from build123d import *

# Parameters (mm, degrees)
PAD018_DEPTH    = 8.5
FILLET008_R     = 6
FILLET009_R     = 3
SKETCH032_R     = 84.3
POCKET021_DEPTH = 9.6
SKETCH033_R     = 1
POCKET022_DEPTH = 17.001
FILLET010_R     = 6


with BuildPart() as part:
    # Sketch031 → Pad018 (new body, symmetric)
    with BuildSketch(Plane.XY):
        with BuildLine():
            Line((226.925203, 42.33455), (276.925203, 128.93709))
            ThreePointArc((310.700194, 109.43709), (294.5, 120.377531), (276.925203, 128.93709))
            Line((260.700194, 22.83455), (310.700194, 109.43709))
            Line((226.925203, 42.33455), (260.700194, 22.83455))
        make_face()
        with BuildLine():
            Line((259.708266, 93.11648), (278.208266, 125.15942))
            ThreePointArc((306.787104, 108.65942), (293, 117.779455), (278.208266, 125.15942))
            Line((288.287104, 76.61648), (306.787104, 108.65942))
            ThreePointArc((288.287104, 76.61648), (274.687379, 86.061065), (259.708266, 93.11648))
        make_face(mode=Mode.SUBTRACT)
    extrude(amount=PAD018_DEPTH, both=True)

    # Fillet008
    fillet008_edges = [part.edges().sort_by_distance(p)[0] for p in [
        (310.700194, 109.43709, 0),
        (276.925203, 128.93709, 0),
    ]]
    fillet(fillet008_edges, radius=FILLET008_R)

    # Fillet009
    fillet009_edges = [part.edges().sort_by_distance(p)[0] for p in [
        (278.208266, 125.15942, 0),
        (306.787104, 108.65942, 0),
    ]]
    fillet(fillet009_edges, radius=FILLET009_R)

    # Sketch032 (on Face1 of Fillet009) → Pocket021 (cut)
    with BuildSketch(Plane(origin=(0, 0, -8.5), x_dir=(1, 0, 0), z_dir=(0, 0, -1))):
        with Locations((225, 0)):
            Circle(SKETCH032_R)
    extrude(amount=-POCKET021_DEPTH, mode=Mode.SUBTRACT)

    # Sketch033 (on Face15 of Pocket021) → Pocket022 (cut, through all)
    with BuildSketch(Plane.XY.offset(8.5)):
        with Locations((245.585457, 54.655058)):
            Circle(SKETCH033_R)
        with Locations((262.03994, 45.155058)):
            Circle(SKETCH033_R)
    extrude(amount=-POCKET022_DEPTH, mode=Mode.SUBTRACT)

    # Fillet010
    fillet010_edges = [part.edges().sort_by_distance(p)[0] for p in [
        (226.925203, 42.33455, 4.8),
        (260.700194, 22.83455, 4.8),
    ]]
    fillet(fillet010_edges, radius=FILLET010_R)


solid = part.part
Can you work these out from the model? Positions are in its coordinate system, mm. A direction names the side the tool comes from. Coordinates: 2 decimals unless noted, no trailing zeros. Write each loop counter-clockwise with the first axis right and the second up, starting at its lowest first coordinate (ties: lowest second). Pieces come first, ordered by that corner, then holes. Notation, with made-up numbers: (60, -18) - (94, -18) arc R29 cw to (94, 14) - close; hole circle Ø11 at (86.25, -40). An arc over 180 degrees is marked (long way). Return JSON: item names as keys, results as strings. Group by question number.
Item 1: Please list where these lines run through material, in increasing order: probe 1 along Z at (x, y) = (252.5, 77); probe 2 along X at (y, z) = (119, 7.75); probe 3 along Y at (x, z) = (285, -6.75).
Item 2: Which directions (+Z, -Z, +X, -X, +Y, -Y) give clear straight access to the entire face, cutting with the end or side of a thin tool? Please do faces 1 (the face through (266.911, 73.143, -3.767)), 2 (the face through (256.714, 93.93, 2.008)), 3 (the face through (296.746, 91.268, 0.119)).
Item 3: If we section it at A-A (z = -3.5): Write out the boundary of the cut face in (x, y), then the cut area to 3 significant figures.
Item 4: I'm going to push flat-ended pins straight in: pin 1 Ø3 at (x, z) = (254, 4.5) entering from +Y; pin 2 Ø3 at (y, z) = (58, 3.5) entering from +X; pin 3 Ø4 at (x, z) = (297, 4.5) entering from +Y. Where does each tip first touch, or does it pass through?
Item 5: If we section it at B-B (x = 284.5): Write out the boundary of the cut face in (y, z).
Item 6: If we section it at D-D (z = 6.25): Write out the boundary of the cut face in (x, y).
Item 7: If we section it at C-C (y = 98.5): Write out the boundary of the cut face in (x, z).
Item 8: We'd pull the mould along Y, two halves only. Please class faces 4 (the face through (260.121, 25.253, 4.852)), 5 (the face through (268.17, 107.77, 0.12)), 6 (the face through (256, 53, 1.1)), 7 (the face through (294.67, 120.28, 0.12)): pulls with the +Y half, pulls with the -Y half, needs draft (parallel to the pull), parting line crosses it, or undercut.
Return value:
{
 "1": {"probe 1": "z = 1.1 to 8.5", "probe 2": "x = 271.19 to 274.65, 290.84 to 296.83", "probe 3": "y = 64.92 to 79.22, 122.05 to 125.38"},
 "2": {"face 1": "-Z, -X, -Y", "face 2": "+Z, -Z, -X, +Y", "face 3": "+Z, -Z"},
 "3": {"outline": "(249.12, 80.78) arc R84.3 cw to (282.89, 61.28) - (308.04, 104.84) arc R6 ccw to (306.36, 112.7) arc R139 ccw to (281.92, 126.81) arc R6 ccw to (274.27, 124.34) - close; hole (259.71, 93.12) arc R99.37 cw to (288.29, 76.62) - (305.45, 106.34) arc R3 ccw to (304.6, 110.27) arc R136 ccw to (280.69, 124.07) arc R3 ccw to (276.87, 122.84) - close", "area": "924 mm^2"},
 "4": {"pin 1": "stops at y = 91.83", "pin 2": "stops at x = 281.87", "pin 3": "stops at y = 120.09"},
 "5": {"outline": "(64.06, -8.5) - (79.59, -8.5) - (79.59, 8.5) - (64.06, 8.5) - close; (122.29, -8.5) - (125.62, -8.5) - (125.62, 8.5) - (122.29, 8.5) - close"},
 "6": {"outline": "(229.93, 47.53) arc R6 ccw to (232.12, 39.33) - (255.5, 25.83) arc R6 ccw to (263.7, 28.03) - (308.04, 104.84) arc R6 ccw to (306.36, 112.7) arc R139 ccw to (281.92, 126.81) arc R6 ccw to (274.27, 124.34) - close; hole circle Ø2 at (245.59, 54.66); hole (259.71, 93.12) arc R99.37 cw to (288.29, 76.62) - (305.45, 106.34) arc R3 ccw to (304.6, 110.27) arc R136 ccw to (280.69, 124.07) arc R3 ccw to (276.87, 122.84) - close; hole circle Ø2 at (262.04, 45.16)"},
 "7": {"outline": "(259.35, -8.5) - (262.82, -8.5) - (262.82, 8.5) - (259.35, 8.5) - close; (300.92, -8.5) - (304.39, -8.5) - (304.39, 8.5) - (300.92, 8.5) - close"},
 "8": {"face 4": "pulls with the -Y half", "face 5": "undercut", "face 6": "needs draft", "face 7": "pulls with the +Y half"}
}
